CAD build for the part. Positions are in the model's coordinates, mm. A direction names the side the tool comes from. Give positions to 0.01 mm unless a question says otherwise; leave off trailing zeros. Write each loop counter-clockwise with the first axis right and the second up, starting at its lowest first coordinate (ties: lowest second). Pieces come first, ordered by that corner, then holes. Notation, with made-up numbers: (73, 27) -> (117, 27) arc R27 cw to (117, 46) -> close; hole circle Ø3 at (15.25, 35). An arc over 180 degrees is marked (long way). Answer in a Markdown table with one row per item. Add a question column.
```python
from build123d import *

# Parameters (mm, degrees)
SKETCH_1_R               = 9
SKETCH_1_R_2             = 4
EXTRUDE_1_DEPTH          = 11
CUT_EXTRUDE_1_OUTLINE_R  = 1.3
CUT_EXTRUDE_1_DEPTH      = 11
PATTERN_CIRCULAR_1_COUNT = 4
CUT_EXTRUDE_2_DEPTH      = 17.822603841


# Read off the part's stored shape, not the designer's step: 切除-拉伸1
with BuildPart() as part:
    # 草图1 → 凸台-拉伸1 (new body)
    with BuildSketch(Plane.XY):
        Circle(SKETCH_1_R)
        Circle(SKETCH_1_R_2, mode=Mode.SUBTRACT)
    extrude(amount=EXTRUDE_1_DEPTH)

    # 切除-拉伸1 outline → 切除-拉伸1 (cut)
    with BuildSketch(Plane.XY):
        with Locations((0, 6.5)):
            Circle(CUT_EXTRUDE_1_OUTLINE_R)
    cut_extrude_1 = extrude(amount=CUT_EXTRUDE_1_DEPTH, mode=Mode.SUBTRACT)

    # 阵列(圆周)1: 切除-拉伸1 ×4 about axis
    pattern_circular_1_axis = Axis((0, 0, 0), (0, 0, 1))
    for i in range(1, PATTERN_CIRCULAR_1_COUNT):
        add(cut_extrude_1.rotate(pattern_circular_1_axis, i * 360 / PATTERN_CIRCULAR_1_COUNT), mode=Mode.SUBTRACT)

    # 草图6 → 切除-拉伸2 (cut, through all)
    with BuildSketch(Plane(origin=(0, 0, 0), x_dir=(-1, 0, 0), z_dir=(0, 0, -1))):
        with BuildLine():
            Line((-4.248676402, 7.934024756), (0, 0))
            Line((0, 0), (-3.930859643, 8.096193085))
            ThreePointArc((-3.930859643, 8.096193085), (-4.090571735, 8.016684033), (-4.248676402, 7.934024756))
        make_face()
    extrude(amount=-CUT_EXTRUDE_2_DEPTH, mode=Mode.SUBTRACT)


solid = part.part
```
Item 1: Slice it at C-C, the plane y = -6.5. List the corners of the cut face in (x, z).
Item 2: Probe L1, parallel to X at y = 0, z = 6.5; L2, parallel to X at y = 6, z = 6.75. List the from-to ranges inside material, lowest first. Write a range as from..to.
Item 3: Slice it at D-D, the plane y = 0.75. List the corners of the cut face in (x, z).
Item 4: Slice it at A-A, the plane x = 0. List the corners of the cut face in (y, z).
Item 5: Mould opens along X. For faces 3 (the face through (3.085, 5.761, 5.423)), 4 (the face through (4, -2, 11)) say: released by +X, released by -X, zero draft, split by the parting line, or undercut.
Item 6: Slice it at B-B, the plane z = 0.5. List the corners of the cut face in (x, y).
Item 7: Which spindle directions (+Z, -Z, +X, -X, +Y, -Y) get a long thin tool onto all of the face, cutting with end or side? Do faces 1 (the face through (4, -2, 0)), 2 (the face through (2.824, 5.816, 5.423)). Say none if no direction does.
Item 8: Drop flat-ended pins along their axis: pin 1 Ø3 at (x, z) = (5.5, 5.5) entering from +Y; pin 2 Ø4 at (x, z) = (5.5, 5) entering from +Y. Give the stop position or say it passes through.
Answer key:
| question | item | result |
|---|---|---|
| 1 | outline | (-6.22, 0) -> (-1.3, 0) -> (-1.3, 11) -> (-6.22, 11) -> close; (1.3, 0) -> (6.22, 0) -> (6.22, 11) -> (1.3, 11) -> close |
| 2 | L1 | x = -9..-7.8, -5.2..-4, 4..5.2, 7.8..9 |
| 2 | L2 | x = -6.71..-1.2, 1.2..2.91, 3.21..6.71 |
| 3 | outline | (-8.97, 0) -> (-7.56, 0) -> (-7.56, 11) -> (-8.97, 11) -> close; (-5.44, 0) -> (-3.93, 0) -> (-3.93, 11) -> (-5.44, 11) -> close; (3.93, 0) -> (5.44, 0) -> (5.44, 11) -> (3.93, 11) -> close; (7.56, 0) -> (8.97, 0) -> (8.97, 11) -> (7.56, 11) -> close |
| 4 | outline | (-9, 0) -> (-7.8, 0) -> (-7.8, 11) -> (-9, 11) -> close; (-5.2, 0) -> (-4, 0) -> (-4, 11) -> (-5.2, 11) -> close; (4, 0) -> (5.2, 0) -> (5.2, 11) -> (4, 11) -> close; (7.8, 0) -> (9, 0) -> (9, 11) -> (7.8, 11) -> close |
| 5 | face 3 | undercut |
| 5 | face 4 | zero draft |
| 6 | outline | (1.75, 3.6) -> (3.93, 8.1) arc R9 ccw (long way) to (4.25, 7.93) -> (1.89, 3.53) arc R4 cw (long way) to start; hole circle Ø2.6 at (-6.5, 0); hole circle Ø2.6 at (0, -6.5); hole circle Ø2.6 at (0, 6.5); hole circle Ø2.6 at (6.5, 0) |
| 7 | face 1 | -Z, +X, -X, +Y, -Y |
| 7 | face 2 | +Z, -Z |
| 8 | pin 1 | stops at y = 7.93 |
| 8 | pin 2 | stops at y = 8.29 |
